Autodesk Inventor part; units mm, degrees
ref_plane "YZ Plane" through (0, 0, 0) normal (1, 0, 0) x (0, 1, 0)
ref_plane "XZ Plane" through (0, 0, 0) normal (0, 1, 0) x (-1, 0, 0)
ref_plane "XY Plane" through (0, 0, 0) normal (0, 0, 1) x (1, 0, 0)
sketch "スケッチ1" plane through (0, 0, 0) normal (0, 0, 1) x (1, 0, 0)
  circle A0 centre (132.465, 0) radius 1.5
  circle A1 centre (45, 0) radius 1.5
  circle A2 centre (102.465, 0) radius 1.5
  circle A3 centre (72.465, 0) radius 1.5
  circle A4 centre (15, 0) radius 1.5
  circle A5 centre (30, 0) radius 1.5
  circle A6 centre (87.465, 0) radius 1.5
  circle A7 centre (117.465, 0) radius 1.5
  circle A8 centre (60, 0) radius 1.5
  circle A9 centre (0, 0) radius 1.5
  line L0 (132.482, -4.5) -> (0.0189, -5)
  arc A10 (0.0189, 5) -> (0.0189, -5) centre (0, 0) ccw
  line L1 (0.0189, 5) -> (132.482, 4.5)
  arc A11 (132.482, -4.5) -> (132.482, 4.5) centre (132.465, 0) ccw
  circle A12 centre (117.465, 0) radius 4.5566
  line L2 (135.2384, -3.5437) -> (160.3015, 16.0714)
  circle A13 centre (132.465, 0) radius 4.5
  line L3 (130.7828, 4.1737) -> (160.3015, 16.0714)
  circle A14 centre (154.1156, 12.5) radius 1
  point P0 (117.4822, -4.5566)
  point P1 (154.732, 11.7125)
  point P2 (153.7418, 13.4275)
  point P3 (131.6004, 4.5033)
  point P4 (117.4822, 4.5566)
  dimension "d0" = 2
  dimension "d1" = 25
  dimension "d2" = 150
extrude "押し出し1" add sketch "スケッチ1" against normal blind 5 contours A13 A11 | L0 A12 L1 L3 A13 | A12 | A11 L1 L3 A14 L2 | L3 L1 A13 | A14
fillet "フィレット1" radius 1 1 edges at (131.6004, 4.5033, -2.5)
sketch "スケッチ2" plane through (0, 0, 0) normal (0, 0, 1) x (1, 0, 0)
  circle A0 centre (117.465, 0) radius 1.5
  circle A1 centre (132.465, 0) radius 1.5
  line L0 (132.482, -4.5) -> (117.4822, -4.5566)
  arc A2 (117.4822, 4.5566) -> (117.4822, -4.5566) centre (117.465, 0) ccw
  line L1 (117.4822, 4.5566) -> (131.4045, 4.504)
  arc A3 (131.4045, 4.504) -> (131.7821, 4.5765) centre (131.4083, 5.504) ccw
  line L2 (131.7821, 4.5765) -> (153.7418, 13.4275)
  arc A4 (154.732, 11.7125) -> (153.7418, 13.4275) centre (154.1156, 12.5) ccw
  line L3 (154.732, 11.7125) -> (135.2384, -3.5437)
  arc A5 (132.482, -4.5) -> (135.2384, -3.5437) centre (132.465, 0) ccw
  line L4 (131.3932, 1.5041) -> (117.4709, 1.5566)
  arc A6 (117.4709, 1.5566) -> (117.4709, -1.5566) centre (117.465, 0) ccw
  line L5 (117.4709, -1.5566) -> (132.4707, -1.5)
  arc A7 (132.4707, -1.5) -> (133.3895, -1.1812) centre (132.465, 0) ccw
  line L6 (133.3895, -1.1812) -> (141.7438, 5.3571)
  line L7 (141.7438, 5.3571) -> (132.9036, 1.794)
  arc A8 (131.3932, 1.5041) -> (132.9036, 1.794) centre (131.4083, 5.504) ccw
  circle A9 centre (117.465, 0) radius 4.5
  circle A10 centre (132.465, 0) radius 4.5
  circle A11 centre (136.965, 2.8567) radius 1
  point P0 (0, 0)
  point P1 (128.2281, -1.516)
  point P2 (128.2281, 1.516)
  point P3 (121.693, 1.5407)
  point P4 (121.693, -1.5407)
  dimension "d6" = 3
  dimension "d7" = 3
  dimension "d8" = 3
  dimension "d9" = 2
extrude "押し出し2" cut sketch "スケッチ2" against normal blind 4.5 contours L5 A9 L4 A10
fillet "フィレット2" radius 1 4 edges at (121.693, 1.5407, -2.25) (121.693, -1.5407, -2.25) (128.2281, 1.516, -2.25) (128.2281, -1.516, -2.25)
properties part number "カウンター 先端部" material "ポリカーボネート、クリア"
Verification items for the finished model (mm, model axes). A direction names the side the tool comes from. Round coordinates to 2 decimals unless told otherwise and drop trailing zeros. Loops run counter-clockwise (first coordinate to the right, second up) from the corner with the lowest first, then second, coordinate; pieces in that order, holes last. Notation, with made-up numbers: (-29, 14.5) - (1, 14.5) arc R22 ccw to (1, 53.5) - close; hole circle Ø9 at (-24, 28). An arc over 180 degrees is marked (long way). Write item = value, one per line.
Q1. Sectioned sample at C-C on z = -3.1. State how many separate pieces and enclosed holes the cut face has, plus the area to 3 significant figures.
Here are the results:
separate_pieces = 1
enclosed_holes = 3
area = 277 mm^2
Q2. Mould release check, pull along Z, two halves, no side actions. Record for faces 3 (the cylindrical face through (127.965, 0.006, -2.218)), 4 (the flat face through (134, 3, -5)), 5 (the flat face through (134, 3, 0)): +Z half, -Z half, draft (parallel to the pull), parting line (faces both ways), or undercut.
Here are the results:
face_3 = draft
face_4 = -Z half
face_5 = +Z half
Q3. Tool access check on faces 1 (the flat face through (142.61, 8.94, -2.46)), 2 (the cylindrical face through (127.74, -1.18, -2.28)). Record the directions out of +Z, -Z, +X, -X, +Y, -Y that give a thin tool (end or side, any length) a straight path to the whole face; none if there is none.
Here are the results:
face_1 = +Z, -Z, -X, +Y
face_2 = +Z
Q4. Sectioned sample at D-D on y = 10.5. Record the boundary of the cut face in (x, z).
Here are the results:
outline = (146.48, -5) - (153.18, -5) - (153.18, 0) - (146.48, 0) - close
Q5. Sectioned sample at A-A on y = 0. Record the boundary of the cut face in (x, z) (3 decimals), plus the area to 3 significant figures.
Here are the results:
outline = (112.908, -5) - (115.965, -5) - (115.965, 0) - (112.908, 0) - close; (118.965, -5) - (130.965, -5) - (130.965, 0) - (127.965, 0) - (127.965, -4.5) - (121.965, -4.5) - (121.965, 0) - (118.965, 0) - close; (133.965, -5) - (139.766, -5) - (139.766, 0) - (133.965, 0) - close
area = 77.3 mm^2
Q6. Material ranges on L1, parallel to X at y = 0.5, z = -0.75; L2, parallel to Y at x = 117, z = -3.75; L3, parallel to Z at x = 125, y = -0.75, recorded low to high.
Here are the results:
L1 = 112.94 to 116.05, 118.88 to 121.94, 127.99 to 131.05, 133.88 to 140.41
L2 = -4.53 to -1.43, 1.43 to 4.53
L3 = -5 to -4.5
Q7. Depth check by flat-ended pin: pin 1 (1.8 mm diameter, centred on x = 117.465, y = 0, fed in from +Z); pin 2 (3 mm diameter, centred on y = 7.5, z = -2.5, fed in from +X); pin 3 (2.5 mm diameter, centred on x = 126, y = 0, fed in from +Z). Enter the tip coordinate at first touch or a pass-through.
Here are the results:
pin_1 = through
pin_2 = 151.27
pin_3 = -4.5
Q8. Sectioned sample at B-B on x = 117. Record the boundary of the cut face in (y, z).
Here are the results:
outline = (-4.53, -5) - (-1.43, -5) - (-1.43, 0) - (-4.53, 0) - close; (1.43, -5) - (4.53, -5) - (4.53, 0) - (1.43, 0) - close
